Model file for the job. Use its own axes, mm. Face numbers are marked on the shaded views. Give positions to 0.01 mm unless a question says otherwise; leave off trailing zeros. Order: outer loops, then holes, each group sorted by start corner. A loop starts at its lowest first (then second) coordinate and runs counter-clockwise, first axis right, second up. Notation, with made-up numbers: (14.5, 32.5) - (40.5, 32.5) arc R23 cw to (40.5, 47.5) - close; hole circle Ø9 at (-4, 70.5). An arc over 180 degrees is marked (long way). Return JSON: item names as keys, results as strings. Group by question number.
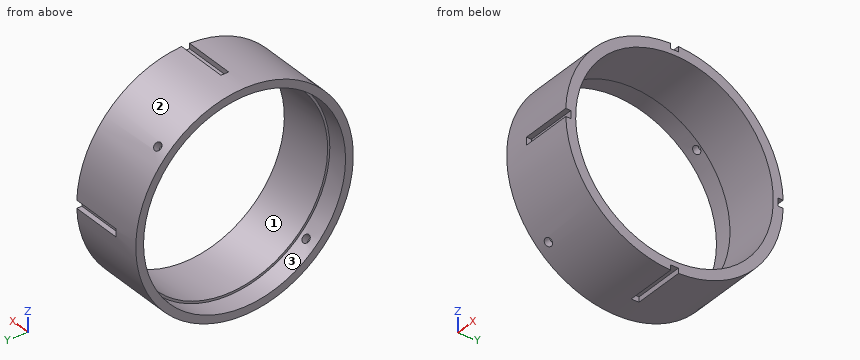
from build123d import *

# Parameters (mm, degrees)
ESQUISSE1_W                  = 30
ESQUISSE1_H                  = 3.85
D_GAGEMENT_M2_51_D           = 3.1
R_P_TITION_CIRCULAIRE1_COUNT = 2
R_P_TITION_CIRCULAIRE1_ANGLE = 90
ESQUISSE4_W                  = 3
ESQUISSE4_H                  = 15
ENL_V_MAT_EXTRU_1_DEPTH      = 20
R_P_TITION_START             = 10
R_P_TITION_CIRCULAIRE2_DEPTH = 20
ESQUISSE5_R                  = 39
ENL_V_MAT_EXTRU_2_DEPTH      = 8


# Read off the part's stored shape, not the designer's step: Répétition circulaire2
with BuildPart() as part:
    # Esquisse1 → Révolution1 (revolve)
    with BuildSketch(Plane.XY, mode=Mode.PRIVATE) as r_volution1_sk:
        with Locations((15, 40.075)):
            Rectangle(ESQUISSE1_W, ESQUISSE1_H)
    revolve(r_volution1_sk.sketch.rotate(Axis((0, 0, 0), (1, 0, 0)), 90), axis=Axis((0, 0, 0), (1, 0, 0)))

    # Dégagement M2.51 (through all)
    with Locations(Plane(origin=(5, -29.69848481, -29.69848481), x_dir=(0, -0.707106781187, 0.707106781187), z_dir=(0, -0.707106781187, -0.707106781187))):
        with Locations((0, 0)):
            d_gagement_m2_51 = Hole(D_GAGEMENT_M2_51_D / 2)

    # Répétition circulaire1: Dégagement M2.51 ×2 about axis
    r_p_tition_circulaire1_axis = Axis((0, 0, 0), (-1, 0, 0))
    for i in range(1, R_P_TITION_CIRCULAIRE1_COUNT):
        add(d_gagement_m2_51.rotate(r_p_tition_circulaire1_axis, i * R_P_TITION_CIRCULAIRE1_ANGLE / (R_P_TITION_CIRCULAIRE1_COUNT - 1)), mode=Mode.SUBTRACT)

    # Esquisse4 → Enlèv. mat.-Extru.1 (cut)
    with BuildSketch(Plane(origin=(30, 0, 0), x_dir=(0, 0, -1), z_dir=(1, 0, 0))):
        with Locations((0, -47.5)):
            Rectangle(ESQUISSE4_W, ESQUISSE4_H)
    extrude(amount=-ENL_V_MAT_EXTRU_1_DEPTH, mode=Mode.SUBTRACT)

    # Répétition circulaire2 outline → Répétition circulaire2 (cut)
    with BuildSketch(Plane.YZ.offset(R_P_TITION_START)):
        with BuildLine():
            ThreePointArc((41.973205739, -1.5), (42, 0), (41.973205739, 1.5))
            Line((41.973205739, 1.5), (40, 1.5))
            Line((40, 1.5), (40, -1.5))
            Line((40, -1.5), (41.973205739, -1.5))
        make_face()
        with BuildLine():
            Line((1.5, 40), (1.5, 41.973205739))
            ThreePointArc((1.5, 41.973205739), (0, 42), (-1.5, 41.973205739))
            Line((-1.5, 41.973205739), (-1.5, 40))
            Line((-1.5, 40), (1.5, 40))
        make_face()
        with BuildLine():
            ThreePointArc((-1.5, -41.973205739), (0, -42), (1.5, -41.973205739))
            Line((1.5, -41.973205739), (1.5, -40))
            Line((1.5, -40), (-1.5, -40))
            Line((-1.5, -40), (-1.5, -41.973205739))
        make_face()
    extrude(amount=R_P_TITION_CIRCULAIRE2_DEPTH, mode=Mode.SUBTRACT)

    # Esquisse5 → Enlèv. mat.-Extru.2 (cut)
    with BuildSketch(Plane.ZY):
        Circle(ESQUISSE5_R)
    extrude(amount=-ENL_V_MAT_EXTRU_2_DEPTH, mode=Mode.SUBTRACT)


solid = part.part
(1) Drill centre lines: L1, parallel to Y at x = 13, z = 0; L2, parallel to Y at x = 23, z = 17; L3, parallel to Z at x = 2.5, y = 18. Where is each one in solid material? Low to high.
(2) Drop flat-ended pins along their axis: pin 1 Ø2.5 at (x, z) = (24, 0) entering from +Y; pin 2 Ø1 at (x, z) = (16, -26.5) entering from +Y; pin 3 Ø3.5 at (x, z) = (21, 0.5) entering from -Y. Give the stop position or say it passes through.
(3) Slice it at B-B (x = 21). Give the cut face in (y, z), and give its area (3 significant figures).
(4) Slice it at D-D (y = 11). Give the cut face in (x, z).
(5) Slice it at A-A (y = 0). Give the cut face in (x, z).
(6) Pull direction Y, two halves, no side cores. Call the marked faces 1, 2 and 3: released by +Y, released by -Y, zero draft, split by the parting line, or undercut.
Result set:
{
 "1": {"L1": "y = -40 to -38.15, 38.15 to 40", "L2": "y = -38.41 to -34.15, 34.15 to 38.41", "L3": "z = -37.95 to -34.6, 34.6 to 37.95"},
 "2": {"pin 1": "stops at y = 40", "pin 2": "stops at y = 32.98", "pin 3": "stops at y = -41.97"},
 "3": {"outline": "(-41.97, -1.5) arc R42 ccw to (-1.5, -41.97) - (-1.5, -40) - (1.5, -40) - (1.5, -41.97) arc R42 ccw to (41.97, -1.5) - (40, -1.5) - (40, 1.5) - (41.97, 1.5) arc R42 ccw to (1.5, 41.97) - (1.5, 40) - (-1.5, 40) - (-1.5, 41.97) arc R42 ccw to (-41.97, 1.5) - (-40, 1.5) - (-40, -1.5) - close; hole circle Ø76.3 at (0, 0)", "area": "946 mm²"},
 "4": {"outline": "(0, -40.53) - (30, -40.53) - (30, -36.53) - (8, -36.53) - (8, -37.42) - (0, -37.42) - close; (0, 37.42) - (8, 37.42) - (8, 36.53) - (30, 36.53) - (30, 40.53) - (0, 40.53) - close"},
 "5": {"outline": "(0, -42) - (10, -42) - (10, -40) - (30, -40) - (30, -38.15) - (8, -38.15) - (8, -39) - (0, -39) - close; (0, 39) - (8, 39) - (8, 38.15) - (30, 38.15) - (30, 40) - (10, 40) - (10, 42) - (0, 42) - close"},
 "6": {"face 1": "undercut", "face 2": "split by the parting line", "face 3": "undercut"}
}
